Autodesk Inventor part; units mm, degrees
ref_plane "YZ Plane" through (0, 0, 0) normal (1, 0, 0) x (0, 1, 0)
ref_plane "XZ Plane" through (0, 0, 0) normal (0, 1, 0) x (-1, 0, 0)
ref_plane "XY Plane" through (0, 0, 0) normal (0, 0, 1) x (1, 0, 0)
sketch "スケッチ1" plane through (0, 0, 0) normal (0, 0, 1) x (1, 0, 0)
  line L0 (0, 0) -> (43.3, 0)
  line L1 (43.3, 28) -> (0, 28)
  line L2 (0, 14) -> (43.3, 14) construction
  line L3 (43.3, 19) -> (45.3, 19)
  line L4 (45.3, 19) -> (45.3, 9)
  line L5 (45.3, 9) -> (43.3, 9)
  arc A0 (43.3, 21) -> (43.3, 19) centre (43.3, 20) ccw
  arc A1 (43.3, 9) -> (43.3, 7) centre (43.3, 8) ccw
  line L6 (43.3, 0) -> (43.3, 7)
  line L7 (43.3, 21) -> (43.3, 28)
  line L8 (21.65, 28) -> (21.65, 0) construction
  line L9 (0, 19) -> (-2, 19)
  line L10 (-2, 19) -> (-2, 9)
  line L11 (-2, 9) -> (0, 9)
  arc A2 (0, 19) -> (0, 21) centre (0, 20) ccw
  arc A3 (0, 7) -> (0, 9) centre (0, 8) ccw
  line L12 (0, 0) -> (0, 7)
  line L13 (0, 21) -> (0, 28)
  dimension "d0" = 43.3
  dimension "d1" = 28
  dimension "d5" = 10
  dimension "d6" = 2
extrude "押し出し1" add sketch "スケッチ1" along normal blind 5
sketch "スケッチ3" plane through (43.3, 0, 0) normal (1, 0, 0) x (0, 0, -1)
  line L0 (0, 0) -> (-5, 0)
  line L1 (-2.5, 0) -> (-2.5, 28) construction
  line L2 (0, 28) -> (-5, 28)
  line L3 (-2.5, 14) -> (0, 14) construction
  line L4 (0, 9) -> (0, 19)
  point P0 (-2.5, 24)
  point P1 (-2.5, 4)
  dimension "d7" = 20
hole "穴1" at (43.3, 24, 2.5) at (43.3, 4, 2.5) direction (-1, 0, 0) diameter 2.4 depth 8 tip angle 118
sketch "スケッチ4" plane through (0, 21, 0) normal (-1, 0, 0) x (0, 0, 1)
  circle A0 centre (2.5, 3) radius 1.2
  circle A1 centre (2.5, -17) radius 1.2
  circle A2 centre (2.5, -17) radius 1.2
  point P0 (0, -21)
hole "穴2" at (0, 24, 2.5) at (0, 4, 2.5) direction (1, 0, 0) diameter 2.4 depth 8 tip angle 118
sketch "スケッチ5" plane through (0, 0, 0) normal (0, 0, -1) x (-1, 0, 0)
  line L0 (0, 0) -> (-43.3, 0)
  line L1 (-21.65, 0) -> (-21.65, 28) construction
  line L2 (-43.3, 28) -> (0, 28)
  line L3 (-21.65, 8.5) -> (-45.9978, 8.5) construction
  point P0 (-32.15, 2.25)
  point P1 (-11.15, 2.25)
  point P2 (-32.15, 14.75)
  point P3 (-11.15, 14.75)
  dimension "d22" = 21
  dimension "d23" = 12.5
  dimension "d24" = 8.5
hole "穴3" at (32.15, 2.25, 0) at (11.15, 2.25, 0) at (11.15, 14.75, 0) at (32.15, 14.75, 0) direction (0, 0, 1) diameter 2.1 end through all
properties part number "頭_メインフレームセンター" material "アセタール樹脂、黒"
Read the model definition and answer for the solid it produces. Units are mm, in the model's axes. A direction names the side the tool comes from. Coordinates: 2 decimals unless noted, no trailing zeros. Loops run counter-clockwise (first coordinate to the right, second up) from the corner with the lowest first, then second, coordinate; pieces in that order, holes last. Notation, with made-up numbers: (39.25, 35) - (73.25, 35) arc R13 ccw to (73.25, 57) - close; hole circle Ø6 at (-3, 48). An arc over 180 degrees is marked (long way). Answer in a Markdown table with one row per item.
Q1. Find section D-D on z = 0.85. Write down the section's boundary in (x, y).
Here are the results:
| item | result |
|---|---|
| outline | (-2, 9) - (0, 9) arc R1 cw to (0, 7) - (0, 0) - (43.3, 0) - (43.3, 7) arc R1 cw to (43.3, 9) - (45.3, 9) - (45.3, 19) - (43.3, 19) arc R1 cw to (43.3, 21) - (43.3, 28) - (0, 28) - (0, 21) arc R1 cw to (0, 19) - (-2, 19) - close; hole circle Ø2.1 at (11.15, 2.25); hole circle Ø2.1 at (11.15, 14.75); hole circle Ø2.1 at (32.15, 2.25); hole circle Ø2.1 at (32.15, 14.75) |
Q2. Find section B-B on y = 2.25. Write down the section's boundary in (x, z), plus the area to 4 significant figures.
Here are the results:
| item | result |
|---|---|
| outline | (0, 0) - (10.1, 0) - (10.1, 5) - (0, 5) - close; (12.2, 0) - (31.1, 0) - (31.1, 5) - (12.2, 5) - close; (33.2, 0) - (43.3, 0) - (43.3, 5) - (33.2, 5) - close |
| area | 195.5 mm^2 |
Q3. Find section C-C on x = 41.5. Write down the section's boundary in (y, z), plus the area to 3 significant figures.
Here are the results:
| item | result |
|---|---|
| outline | (0, 0) - (28, 0) - (28, 5) - (0, 5) - close; hole circle Ø2.4 at (4, 2.5); hole circle Ø2.4 at (24, 2.5) |
| area | 131 mm^2 |
Q4. The mould has two halves that part along Y. Classify faces 1 (the cylindrical face through (39.244, 25.065, 1.946)), 2 (the flat face through (21, 14, 0)), 3 (the flat face through (44, 9, 2)), 4 (the flat face through (44, 19, 2)): pulls with the +Y half, pulls with the -Y half, needs draft (parallel to the pull), parting line crosses it, or undercut.
Here are the results:
| item | result |
|---|---|
| face 1 | undercut |
| face 2 | needs draft |
| face 3 | pulls with the -Y half |
| face 4 | pulls with the +Y half |
Q5. Straight lines are drawn through the part: line 1 along X through (y, z) = (14.75, 2); line 2 along X through (y, z) = (2.25, 2.7); line 3 along Y through (x, z) = (32.15, 1.7). For each, find the intervals that lie inside material, in ascending order. Write a range as [from, to].
Here are the results:
| item | result |
|---|---|
| line 1 | x = [-2, 10.1], [12.2, 31.1], [33.2, 45.3] |
| line 2 | x = [0, 10.1], [12.2, 31.1], [33.2, 43.3] |
| line 3 | y = [0, 1.2], [3.3, 13.7], [15.8, 28] |
Q6. For faces 5 (the cylindrical face through (39.244, 3.64, 1.355)), 6 (the cylindrical face through (4.06, 4.46, 3.61)), 7 (the flat face through (-1, 9, 2)), 8 (the flat face through (43.3, 2.7, 1.9)), determine the directions among +Z, -Z, +X, -X, +Y, -Y from which every point of the face is accessible in a straight line to the end or side of a thin tool.
Here are the results:
| item | result |
|---|---|
| face 5 | +X |
| face 6 | -X |
| face 7 | +Z, -Z, -X, -Y |
| face 8 | +Z, -Z, +X, -Y |
Q7. Given P1, Ø1.3, axis at x = 11.15, y = 14.75, coming from the -Z side; P2, Ø1.9, axis at y = 4, z = 2.5, coming from the -X side; P3, Ø2, axis at x = 45, z = 1.5, coming from the -Y side; P4, Ø0.6, axis at x = 44, z = 2.5, coming from the +Y side, each flat-ended and moving along its own axis, determine where each tip first touches the part or whether it passes through.
Here are the results:
| item | result |
|---|---|
| P1 | passes through |
| P2 | stops at x = 8.15 |
| P3 | stops at y = 9 |
| P4 | stops at y = 19 |
Q8. Find section A-A on x = 32.15. Write down the section's boundary in (y, z).
Here are the results:
| item | result |
|---|---|
| outline | (0, 0) - (1.2, 0) - (1.2, 5) - (0, 5) - close; (3.3, 0) - (13.7, 0) - (13.7, 5) - (3.3, 5) - close; (15.8, 0) - (28, 0) - (28, 5) - (15.8, 5) - close |
